Can you work these out from the model? Positions are in its coordinate system, mm. A direction names the side the tool comes from. Coordinates: 2 decimals unless noted, no trailing zeros. Loops run counter-clockwise (first coordinate to the right, second up) from the corner with the lowest first, then second, coordinate; pieces in that order, holes last.
```python
from build123d import *

# Parameters (mm, degrees)
F0_W     = 76.2
F0_H     = 50.8
F0_R     = 12.7
F1_DEPTH = 25.4
F2_W     = 6.35
F2_H     = 50.8
F3_DEPTH = 2.54
F5_DEPTH = 50.801
F6_R     = 5.6836781625
F7_DEPTH = 25.4


with BuildPart() as f1:
    # F0 (on Front) → F1 (new body)
    with BuildSketch(Plane.XZ):
        Rectangle(F0_W, F0_H)
        Circle(F0_R, mode=Mode.SUBTRACT)
    extrude(amount=F1_DEPTH)

    # F2 (on face) → F3 (cut)
    with BuildSketch(Plane.XZ.offset(25.4)):
        with Locations((-32.385, 0)):
            Rectangle(F2_W, F2_H)
        with BuildLine():
            Line((-5.324405618, -11.5299915358), (-5.324405618, -25.4))
            Line((-5.324405618, -25.4), (4.835594382, -25.4))
            Line((4.835594382, -25.4), (4.835594382, -11.7433822629))
            ThreePointArc((4.835594382, -11.7433822629), (-0.2666795956, -12.6971997698), (-5.324405618, -11.5299915358))
        make_face()
        with BuildLine():
            Line((4.835594382, 25.4), (-5.324405618, 25.4))
            Line((-5.324405618, 25.4), (-5.324405618, 11.5299915358))
            ThreePointArc((-5.324405618, 11.5299915358), (-0.2666795956, 12.6971997698), (4.835594382, 11.7433822629))
            Line((4.835594382, 11.7433822629), (4.835594382, 25.4))
        make_face()
    extrude(amount=-F3_DEPTH, mode=Mode.SUBTRACT)

    # F4 (on face) → F5 (cut, through all)
    with BuildSketch(Plane(origin=(0, 0, -25.4), x_dir=(1, 0, 0), z_dir=(0, 0, -1))):
        Polygon((21.467797191, 25.4), (13.0851396952, 25.4), (10.1522003277, 20.32), (24.4007365585, 20.32), align=None)
    extrude(amount=-F5_DEPTH, mode=Mode.SUBTRACT)

    # F6 (on face) → F7 (join)
    with BuildSketch(Plane.YZ.offset(38.1)):
        with Locations((-13.3386543021, 0)):
            Circle(F6_R)
    extrude(amount=F7_DEPTH)


solid = f1.part
```
(1) I want a section at D-D on z = 16. Write out the boundary of the cut face in (x, y).
Check values:
outline: (-38.1, -25.4) - (-35.56, -25.4) - (-35.56, -22.86) - (-29.21, -22.86) - (-29.21, -25.4) - (-5.32, -25.4) - (-5.32, -22.86) - (4.84, -22.86) - (4.84, -25.4) - (13.09, -25.4) - (10.15, -20.32) - (24.4, -20.32) - (21.47, -25.4) - (38.1, -25.4) - (38.1, 0) - (-38.1, 0) - close
(2) I'm going to push flat-ended pins straight in: pin 1 (1.3 mm diameter, centred on y = -24.5, z = 16, fed in from +X); pin 2 (10 mm diameter, centred on x = 9.5, z = 9.5, fed in from +Y); pin 3 (5 mm diameter, centred on x = 0, z = -21, fed in from -Y); pin 4 (1 mm diameter, centred on x = 45.5, y = -17, fed in from +Z). Where does each tip first touch, or does it pass through?
Check values:
pin 1: stops at x = 38.1
pin 2: stops at y = 0
pin 3: stops at y = -22.86
pin 4: stops at z = 4.72
(3) If we mould it in two halves opening along X, with no side actions, what happens to faces 4 (the flat face through (8, 0, 12)), 5 (the flat face through (-38.1, -13, 0)), 6 (the flat face through (-5.324, -24, -18))? For each: released by +X, released by -X, zero draft, split by the parting line, or undercut.
Check values:
face 4: zero draft
face 5: released by -X
face 6: undercut
(4) I want a section at C-C on y = -13. Write out the boundary of the cut face in (x, z), then the cut area to 3 significant figures.
Check values:
outline: (-38.1, -25.4) - (38.1, -25.4) - (38.1, -5.67) - (63.5, -5.67) - (63.5, 5.67) - (38.1, 5.67) - (38.1, 25.4) - (-38.1, 25.4) - close; hole circle Ø25.4 at (0, 0)
area: 3,650 mm2
(5) I want a section at A-A on x = 0. Write out the boundary of the cut face in (y, z), then the cut area to 3 significant figures.
Check values:
outline: (-22.86, -25.4) - (0, -25.4) - (0, -12.7) - (-22.86, -12.7) - close; (-22.86, 12.7) - (0, 12.7) - (0, 25.4) - (-22.86, 25.4) - close
area: 581 mm2
(6) If I drill on probe 1 along Z at (x, y) = (0, -18.75); probe 2 along X at (y, z) = (-11, 0); probe 3 along X at (y, z) = (-19.75, -15), over which ranges is the centre line in solid material (lowest first)?
Check values:
probe 1: z = -25.4 to -12.7, 12.7 to 25.4
probe 2: x = -38.1 to -12.7, 12.7 to 63.5
probe 3: x = -38.1 to 38.1
(7) Which directions (+Z, -Z, +X, -X, +Y, -Y) give clear straight access to the entire face, cutting with the end or side of a thin tool? Please do faces 1 (the flat face through (12.94, -25.15, -0.36)), 2 (the cylindrical face through (50.6, -8.1, -2.2)), 3 (the flat face through (4.836, -24, -19)).
Check values:
face 1: +Z, -Z
face 2: +X
face 3: +Z, -Z, -Y
(8) I want a section at B-B on z = 0. Write out the boundary of the cut face in (x, y), then the cut area to 3 significant figures.
Check values:
outline: (-38.1, -25.4) - (-35.56, -25.4) - (-35.56, -22.86) - (-29.21, -22.86) - (-29.21, -25.4) - (-12.7, -25.4) - (-12.7, 0) - (-38.1, 0) - close; (12.7, -25.4) - (13.09, -25.4) - (12.7, -24.73) - close; (12.7, -20.32) - (24.4, -20.32) - (21.47, -25.4) - (38.1, -25.4) - (38.1, -19.02) - (63.5, -19.02) - (63.5, -7.65) - (38.1, -7.65) - (38.1, 0) - (12.7, 0) - close
area: 1,510 mm2
